Build history of the part. All positions in model axes, mm. A direction names the side the tool comes from. Coordinates: 2 decimals unless noted, no trailing zeros. Order: outer loops, then holes, each group sorted by start corner. A loop starts at its lowest first (then second) coordinate and runs counter-clockwise, first axis right, second up. Notation, with made-up numbers: M 20,-20 L 54,-20 A20 cw 54,-5 Z; hole C 72.5,47.5 d6. An arc over 180 degrees is marked long. Write item = value, one per line. Start each with the question number.
Q1. 3-axis set-ups, long thin cutter, end or side, ignore diameter. For faces 1 (the face through (126.847, 86.276, 1.479)), 2 (the face through (-124, 89, 0)): which of +Z, -Z, +X, -X, +Y, -Y reach the whole face in a straight line?
Q2. Drill centre lines: probe 1 along Y at (x, z) = (159, 1.9); probe 2 along X at (y, z) = (55, 1); probe 3 along X at (y, z) = (169, 1.9). Where is each one in solid material? Low to high.
Q3. Band-saw the part on B-B on y = -35. Write the cut outline in (x, z), plus the area to 3 significant figures.
Q4. Band-saw the part on C-C on z = 2.2. State how many separate pieces and enclosed holes the cut face has, plus the area to 3 significant figures.
Q5. Band-saw the part on A-A on x = -33.5. Write the cut outline in (y, z).
Q6. Pull direction X, two halves, no side cores. Call faces 3 (the face through (-88.564, 97.994, 1.479)), 4 (the face through (-124, 89, 3)): released by +X, released by -X, zero draft, split by the parting line, or undercut.
```python
from build123d import *

# Parameters (mm, degrees)
SKETCH_W          = 365.0996
SKETCH_H          = 379.984
SKETCH_R          = 5
SKETCH_W_2        = 10.5
SKETCH_H_2        = 3.5
PAD_DEPTH         = 3
POCKET_DEPTH      = 0.001
POCKET_DEPTH_BACK = -3.001


with BuildPart() as part:
    # Sketch → Pad (new body)
    with BuildSketch(Plane.XY):
        with Locations((0, 2.2987)):
            Rectangle(SKETCH_W, SKETCH_H)
        with Locations((-159.9946, 167.2971)):
            Circle(SKETCH_R, mode=Mode.SUBTRACT)
        with Locations((159.9946, 167.2971)):
            Circle(SKETCH_R, mode=Mode.SUBTRACT)
        with Locations((159.9946, -167.2971)):
            Circle(SKETCH_R, mode=Mode.SUBTRACT)
        with Locations((-159.9946, -167.2971)):
            Circle(SKETCH_R, mode=Mode.SUBTRACT)
        with Locations((-140, -132.419)):
            Rectangle(SKETCH_W_2, SKETCH_H_2, mode=Mode.SUBTRACT)
        with Locations((-100, -132.419)):
            Rectangle(SKETCH_W_2, SKETCH_H_2, mode=Mode.SUBTRACT)
        with Locations((100, -132.419)):
            Rectangle(SKETCH_W_2, SKETCH_H_2, mode=Mode.SUBTRACT)
        with Locations((140, -132.419)):
            Rectangle(SKETCH_W_2, SKETCH_H_2, mode=Mode.SUBTRACT)
        with Locations((-162.2998, 114.7971)):
            Rectangle(SKETCH_W_2, SKETCH_H_2, mode=Mode.SUBTRACT)
        with Locations((-122.2998, 114.7971)):
            Rectangle(SKETCH_W_2, SKETCH_H_2, mode=Mode.SUBTRACT)
        with Locations((122.2998, 114.7971)):
            Rectangle(SKETCH_W_2, SKETCH_H_2, mode=Mode.SUBTRACT)
        with Locations((162.2998, 114.7971)):
            Rectangle(SKETCH_W_2, SKETCH_H_2, mode=Mode.SUBTRACT)
    extrude(amount=PAD_DEPTH)

    # Sketch001 → Pocket (cut, two sides)
    with BuildSketch(Plane.XY) as pocket_sk:
        with BuildLine():
            Line((0, 142.2907), (-62.5498, 142.2907))
            ThreePointArc((-62.5498, 142.2907), (-76.691936, 136.432836), (-82.5498, 122.2907))
            Line((-82.5498, 122.2907), (-82.5498, 112.2907))
            ThreePointArc((-102.5498, 92.2907), (-88.407664, 98.148564), (-82.5498, 112.2907))
            Line((-112.5498, 92.2907), (-102.5498, 92.2907))
            ThreePointArc((-112.5498, 92.2907), (-126.691936, 86.432836), (-132.5498, 72.2907))
            Line((-132.5498, 0), (-132.5498, 72.2907))
            Line((-132.5498, 0), (-132.5498, -72.2907))
            ThreePointArc((-132.5498, -72.2907), (-126.691936, -86.432836), (-112.5498, -92.2907))
            Line((-112.5498, -92.2907), (-102.5498, -92.2907))
            ThreePointArc((-82.5498, -112.2907), (-88.407664, -98.148564), (-102.5498, -92.2907))
            Line((-82.5498, -122.2907), (-82.5498, -112.2907))
            ThreePointArc((-82.5498, -122.2907), (-76.691936, -136.432836), (-62.5498, -142.2907))
            Line((0, -142.2907), (-62.5498, -142.2907))
            Line((0, -142.2907), (62.5498, -142.2907))
            ThreePointArc((62.5498, -142.2907), (76.691935, -136.432835), (82.549799, -122.2907))
            Line((82.549799, -122.2907), (82.549799, -112.2907))
            ThreePointArc((102.5498, -92.290701), (88.407664, -98.148564), (82.549799, -112.2907))
            Line((112.5498, -92.290701), (102.5498, -92.290701))
            ThreePointArc((112.5498, -92.290701), (126.691936, -86.432836), (132.5498, -72.2907))
            Line((132.5498, 0), (132.5498, -72.2907))
            Line((132.5498, 0), (132.5498, 72.2907))
            ThreePointArc((132.5498, 72.2907), (126.691936, 86.432836), (112.5498, 92.290701))
            Line((112.5498, 92.290701), (102.5498, 92.290701))
            ThreePointArc((82.549799, 112.2907), (88.407664, 98.148564), (102.5498, 92.290701))
            Line((82.549799, 122.2907), (82.549799, 112.2907))
            ThreePointArc((82.549799, 122.2907), (76.691935, 136.432835), (62.5498, 142.2907))
            Line((0, 142.2907), (62.5498, 142.2907))
        make_face()
    extrude(amount=-POCKET_DEPTH, mode=Mode.SUBTRACT)
    extrude(pocket_sk.sketch, amount=-POCKET_DEPTH_BACK, mode=Mode.SUBTRACT)


solid = part.part
```
Recorded:
q1.face_1 = +Z, -Z
q1.face_2 = -Z, +X, -X, +Y, -Y
q2.probe_1 = -187.69 to -172.2, -162.4 to 113.05, 116.55 to 162.4, 172.2 to 192.29
q2.probe_2 = -182.55 to -132.55, 132.55 to 182.55
q2.probe_3 = -182.55 to -164.7, -155.29 to 155.29, 164.7 to 182.55
q3.outline = M -182.55,0 L -132.55,0 L -132.55,3 L -182.55,3 Z; M 132.55,0 L 182.55,0 L 182.55,3 L 132.55,3 Z
q3.area = 300 mm2
q4.separate_pieces = 1
q4.enclosed_holes = 13
q4.area = 73,000 mm2
q5.outline = M -187.69,0 L -142.29,0 L -142.29,3 L -187.69,3 Z; M 142.29,0 L 192.29,0 L 192.29,3 L 142.29,3 Z
q6.face_3 = undercut
q6.face_4 = zero draft
